```python
from build123d import *

# Parameters (mm, degrees)
BOSS_EXTRUDE1_DEPTH = 15
BOSS_EXTRUDE2_DEPTH = 18
BOSS_EXTRUDE3_DEPTH = 15
SKETCH4_R           = 4.5
CUT_EXTRUDE1_DEPTH  = 15
BOSS_EXTRUDE4_DEPTH = 36
SKETCH6_W           = 12
SKETCH6_H           = 24
CUT_EXTRUDE2_DEPTH  = 61.125389812
SKETCH7_W           = 15
SKETCH7_H           = 10.623328836
BOSS_EXTRUDE5_DEPTH = 36
BOSS_EXTRUDE6_DEPTH = 15


with BuildPart() as part:
    # Sketch1 → Boss-Extrude1 (new body)
    with BuildSketch(Plane(origin=(0, 0, 0), x_dir=(0, 0, -1), z_dir=(1, 0, 0))):
        with BuildLine():
            Line((-25.766620498, 0), (36.265250882, 0))
            Line((36.265250882, 0), (36.265250882, 36))
            Line((36.265250882, 36), (0.265250882, 36))
            Line((0.265250882, 36), (0.265250882, 18))
            Line((0.265250882, 18), (-23.734749118, 18))
            Line((-23.734749118, 18), (-23.734749118, 19.356781067))
            Line((-23.734749118, 19.356781067), (-41.734749118, 19.356781067))
            ThreePointArc((-41.734749118, 19.356781067), (-37.227535866, 6.810206785), (-25.766620498, 0))
        make_face()
    extrude(amount=-BOSS_EXTRUDE1_DEPTH)

    # Sketch2 → Boss-Extrude2 (add)
    with BuildSketch(Plane.XY.offset(23.75)):
        Polygon((-15, 19.356781067), (-23.791342675, 35.356781067), (-23.791342675, 47.356781067), (-8.791342675, 47.356781067), (-8.791342675, 35.356781067), (0, 19.356781067), align=None)
    extrude(amount=BOSS_EXTRUDE2_DEPTH)

    # Sketch3 → Boss-Extrude3 (add)
    with BuildSketch(Plane(origin=(-8.791342675, 0, 0), x_dir=(0, 0, -1), z_dir=(1, 0, 0))):
        with BuildLine():
            Line((-41.75, 47.356781067), (-23.75, 47.356781067))
            ThreePointArc((-23.75, 47.356781067), (-32.75, 56.356781067), (-41.75, 47.356781067))
        make_face()
    extrude(amount=-BOSS_EXTRUDE3_DEPTH)

    # Sketch4 → Cut-Extrude1 (cut)
    with BuildSketch(Plane(origin=(-8.791342675, 0, 0), x_dir=(0, 0, -1), z_dir=(1, 0, 0))):
        with Locations((-32.75, 47.356781067)):
            Circle(SKETCH4_R)
    extrude(amount=-CUT_EXTRUDE1_DEPTH, mode=Mode.SUBTRACT)


with BuildPart() as body_2:
    # Sketch5 → Boss-Extrude4 (new body)
    with BuildSketch(Plane(origin=(0, 36, 0), x_dir=(1, 0, 0), z_dir=(0, 1, 0))):
        Polygon((-15, 36.265250882), (-24, 36.265250882), (-24, 0), (-15, 0.265250882), align=None)
    extrude(amount=-BOSS_EXTRUDE4_DEPTH)


with BuildPart() as cut_extrude2_tool:
    # Sketch6 → Cut-Extrude2 (new, through all)
    with BuildSketch(Plane(origin=(0, 36, 0), x_dir=(1, 0, 0), z_dir=(0, 1, 0))):
        with Locations((-12, 18.265250882)):
            Rectangle(SKETCH6_W, SKETCH6_H)
    extrude(amount=-CUT_EXTRUDE2_DEPTH)


with BuildPart() as part_1:
    add(part.part)

    # Cut-Extrude2: cut by cut_extrude2_tool
    add(cut_extrude2_tool.part, mode=Mode.SUBTRACT)



with BuildPart() as body_2_1:
    add(body_2.part)

    # Cut-Extrude2: cut by cut_extrude2_tool
    add(cut_extrude2_tool.part, mode=Mode.SUBTRACT)


with BuildPart() as part_2:
    add(part_1.part)

    add(body_2_1.part)  # Boss-Extrude5 merges body 2
    # Sketch7 → Boss-Extrude5 (add)
    with BuildSketch(Plane(origin=(0, 36, 0), x_dir=(1, 0, 0), z_dir=(0, 1, 0))):
        with Locations((-10.5, 41.5769153)):
            Rectangle(SKETCH7_W, SKETCH7_H)
    extrude(amount=-BOSS_EXTRUDE5_DEPTH)

    # Sketch9 → Boss-Extrude6 (add)
    with BuildSketch(Plane(origin=(-3, 0, 0), x_dir=(0, 0, -1), z_dir=(1, 0, 0))):
        with BuildLine():
            Line((46.888579718, 76), (46.888579718, 36))
            Line((46.888579718, 36), (46.888579718, 0))
            ThreePointArc((46.888579718, 0), (68.212387297, 10.028536545), (76.888579718, 31.937438845))
            Line((76.888579718, 31.937438845), (76.888579718, 76))
            Line((76.888579718, 76), (62.888579718, 76))
            Line((62.888579718, 76), (62.888579718, 60.94427191))
            ThreePointArc((62.888579718, 60.94427191), (68.59678365, 58), (70.888579718, 52))
            ThreePointArc((70.888579718, 52), (55.888579718, 45.291796068), (60.888579718, 60.94427191))
            Line((60.888579718, 60.94427191), (60.888579718, 76))
            Line((60.888579718, 76), (46.888579718, 76))
        make_face()
    extrude(amount=-BOSS_EXTRUDE6_DEPTH)


solid = part_2.part
```
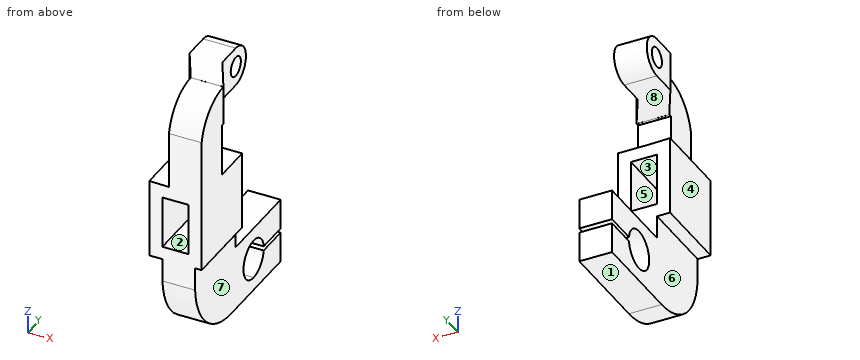
For this review, take the finished solid that the model builds, in its own axes (mm). Face numbers are marked on the shaded views. A direction names the side the tool comes from. Coordinates: 2 decimals unless noted, no trailing zeros. Loops run counter-clockwise (first coordinate to the right, second up) from the corner with the lowest first, then second, coordinate; pieces in that order, holes last.
1. For the marked faces 5, 6, 7 and 8, list the 3-axis set-ups (+Z, -Z, +X, -X, +Y, -Y) from which the entire face can be reached by the end or side of a thin tool; tool diameter is ignored.
2. Mouldability with a two-part tool opening along Z and no side actions: class the marked faces 1, 2, 3 and 4 as +Z half, -Z half, draft (parallel to the pull), parting line (faces both ways), or undercut.
3. Add section D-D, the plane z = 32.75. Give the boundary of the cut face in (x, y), then the cut area to 3 significant figures.
4. Add section B-B, the plane z = -21. Give the boundary of the cut face in (x, y).
5. Add section A-A, the plane y = 40. Give the boundary of the cut face in (x, z), then the cut area to 3 significant figures.
6. For line 1 (Z direction, x = -6.25, y = 52); line 2 (Z direction, x = -15.75, y = 54.5); line 3 (Z direction, x = -4.75, y = 62), list the stretches that pass through material, from the lowest coordinate up.
7. Add section C-C, the plane x = -21.5. Give the boundary of the cut face in (y, z), then the cut area to 3 significant figures.
8. Insertion check: P1, Ø21.5, axis at y = 7.5, z = 31, coming from the -X side; P2, Ø1, axis at x = -5.5, y = 42, coming from the +Z side; P3, Ø3, axis at y = 41.5, z = -52.5, coming from the -X side; P4, Ø5.5, axis at y = 48, z = 31.5, coming from the +X side. Each pin has a flat end and moves straight along its axis. Give the tip position at first contact, or say it passes through.
Result:
1. face 5: +Y, -Y
1. face 6: -Z, -X, +Y, -Y
1. face 7: -Z, +X, +Y, -Y
1. face 8: +X, -X, +Y
2. face 1: -Z half
2. face 2: undercut
2. face 3: undercut
2. face 4: draft
3. outline: (-23.79, 35.36) - (-15, 19.36) - (-15, 2.82) - (0, 2.82) - (0, 19.36) - (-8.79, 35.36) - (-8.79, 42.86) - (-23.79, 42.86) - close; (-23.79, 51.86) - (-8.79, 51.86) - (-8.79, 56.36) - (-23.79, 56.36) - close
3. area: 668 mm2
4. outline: (-24, 0) - (-18, 0) - (-18, 36) - (-24, 36) - close; (-6, 0) - (0, 0) - (0, 36) - (-6, 36) - close
5. outline: (-23.79, 23.75) - (-8.79, 23.75) - (-8.79, 41.75) - (-23.79, 41.75) - close; (-18, -76.89) - (-3, -76.89) - (-3, -46.89) - (-18, -46.89) - close
5. area: 720 mm2
6. line 1: z = -76.89 to -70.89, -52.89 to -46.89
6. line 2: z = -76.89 to -70.53, -53.24 to -46.89, 27.28 to 38.22
6. line 3: z = -76.89 to -62.89, -60.89 to -46.89
7. outline: (0, -36.27) - (36, -36.27) - (36, -0.07) - (0, -0.07) - close; (31.19, 23.75) - (47.36, 23.75) arc R9 ccw to (47.36, 41.75) - (31.19, 41.75) - close; hole circle Ø9 at (47.36, 32.75)
7. area: 1,660 mm2
8. P1: stops at x = -15
8. P2: stops at z = -46.89
8. P3: stops at x = -18
8. P4: passes through
